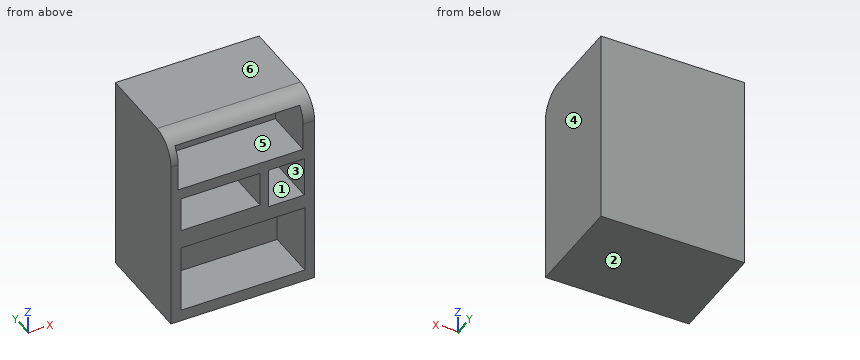
```python
from build123d import *

# Parameters (mm, degrees)
F0_W        = 71.2871104479
F0_H        = 49.0286853164
F0_W_2      = 58.531470614
F0_H_2      = 36.0211754636
F0_W_3      = 60.9135755652
F0_H_3      = 33.0608540971
F1_DEPTH    = 50.8
F2_W        = 39.112127386
F2_H        = 17.2953940928
F2_W_2      = 17.7711145952
F2_H_2      = 19.8306103703
F2_W_3      = 61.416560784
F2_H_3      = 33.9031042531
F2_W_4      = 61.9626361877
F2_H_4      = 21.9576358795
F3_DEPTH    = 25.4
F4_T1_DEPTH = 134.7871104479


# Not quite as in the source:
# - a fillet or chamfer that OpenCascade refuses, or shapes differently, is made with other operations: its cross-section is extruded or revolved along the edge and cut away or added


with BuildPart() as f1:
    # F0 (on Front) → F1 (new body)
    with BuildSketch(Plane.XZ):
        with Locations((0, 24.5143426582)):
            Rectangle(F0_W, F0_H)
        with Locations((-0.6145685997, 23.0905877318)):
            Rectangle(F0_W_2, F0_H_2, mode=Mode.SUBTRACT)
        with Locations((0, -24.5143426582)):
            Rectangle(F0_W, F0_H)
        with Locations((0.2925068763, -25.7660689676)):
            Rectangle(F0_W_3, F0_H_3, mode=Mode.SUBTRACT)
        with Locations((-0.6145685997, 23.0905877318)):
            Rectangle(F0_W_2, F0_H_2)
        with Locations((0.2925068763, -25.7660689676)):
            Rectangle(F0_W_3, F0_H_3)
    extrude(amount=F1_DEPTH)

    # F2 (on face) → F3 (cut)
    with BuildSketch(Plane.XZ.offset(50.8)):
        with Locations((-10.9740667976, 8.6476970464)):
            Rectangle(F2_W, F2_H)
        with Locations((21.669532638, 7.5109825702)):
            Rectangle(F2_W_2, F2_H_2)
        with Locations((0.1781499013, -26.3703963719)):
            Rectangle(F2_W_3, F2_H_3)
        with Locations((-1.0527623817, 33.6884222925)):
            Rectangle(F2_W_4, F2_H_4)
    extrude(amount=-F3_DEPTH, mode=Mode.SUBTRACT)

    # F4: fillet of radius 12.7 on 1 edges, made by hand

    # F4_s2 → F4_t1 (cut)
    with BuildSketch(Plane.YZ.offset(-67.3935552239)):
        with BuildLine():
            ThreePointArc((-50.8, 36.3286853164), (-47.0802561211, 45.3089414375), (-38.1, 49.0286853164))
            Line((-38.1, 49.0286853164), (-50.8, 49.0286853164))
            Line((-50.8, 49.0286853164), (-50.8, 36.3286853164))
        make_face()
    extrude(amount=F4_T1_DEPTH, mode=Mode.SUBTRACT)


solid = f1.part
```
Geometry: final body of the model. Coordinates: model frame, mm. Face numbers are marked on the shaded views. A direction names the side the tool comes from. Round coordinates to 2 decimals unless told otherwise and drop trailing zeros. Order: outer loops, then holes, each group sorted by start corner. A loop starts at its lowest first (then second) coordinate and runs counter-clockwise, first axis right, second up. Notation, with made-up numbers: (3, 3.25) -> (47, 3.25) arc R21 cw to (47, 22.25) -> close; hole circle Ø3 at (49.5, 83). An arc over 180 degrees is marked (long way). Use CSV: the item, a comma, the result in double quotes. Start each with the question number.
1) Section D-D (x = -1). Return the cut outline in (y, z), and give its area (3 significant figures).
2) First-contact query: pin 1 Ø4 at (x, z) = (5.5, 36) entering from -Y. Flat tip, straight axial feed; report the tip coordinate or a pass-through.
3) Section A-A (y = -33.5). Return the cut outline in (x, z), and give its area (3 significant figures).
4) Section B-B (x = 25). Return the cut outline in (y, z).
5) Set-up query: the marked faces 1 and 2. Return all of +Z, -Z, +X, -X, +Y, -Y with unobstructed straight access to the full face (end or side cutting, diameter ignored); none if empty.
6) Section C-C (z = -33.5). Return the cut outline in (x, y).
7) Material intervals for line 1 along Z through (x, y) = (-4, -33); line 2 along X through (y, z) = (-28, 16.5); line 3 along Z through (x, y) = (-32, -31), sorted ascending. Write a range as from..to.
8) Draft query along X for the marked faces 3, 4, 5 and 6. Return one class per face: +X half, -X half, draft (parallel to the pull), parting line (faces both ways), or undercut.
Returned:
1,outline,"(-50.8, -49.03) -> (0, -49.03) -> (0, 49.03) -> (-38.1, 49.03) arc R12.7 ccw to (-47.68, 44.67) -> (-25.4, 44.67) -> (-25.4, 22.71) -> (-50.8, 22.71) -> (-50.8, 17.3) -> (-25.4, 17.3) -> (-25.4, 0) -> (-50.8, 0) -> (-50.8, -9.42) -> (-25.4, -9.42) -> (-25.4, -43.32) -> (-50.8, -43.32) -> close"
1,area,"3,100 mm²"
2,pin 1,"stops at y = -25.4"
3,outline,"(-35.64, -49.03) -> (35.64, -49.03) -> (35.64, 49.03) -> (-35.64, 49.03) -> close; hole (-32.03, 22.71) -> (29.93, 22.71) -> (29.93, 44.67) -> (-32.03, 44.67) -> close; hole (-30.53, -43.32) -> (30.89, -43.32) -> (30.89, -9.42) -> (-30.53, -9.42) -> close; hole (-30.53, 0) -> (8.58, 0) -> (8.58, 17.3) -> (-30.53, 17.3) -> close; hole (12.78, -2.4) -> (30.56, -2.4) -> (30.56, 17.43) -> (12.78, 17.43) -> close"
3,area,"2,520 mm²"
4,outline,"(-50.8, -49.03) -> (0, -49.03) -> (0, 49.03) -> (-38.1, 49.03) arc R12.7 ccw to (-47.68, 44.67) -> (-25.4, 44.67) -> (-25.4, 22.71) -> (-50.8, 22.71) -> (-50.8, 17.43) -> (-25.4, 17.43) -> (-25.4, -2.4) -> (-50.8, -2.4) -> (-50.8, -9.42) -> (-25.4, -9.42) -> (-25.4, -43.32) -> (-50.8, -43.32) -> close"
5,face 1,"-Y"
5,face 2,"-Z, +X, -X, +Y, -Y"
6,outline,"(-35.64, -50.8) -> (-30.53, -50.8) -> (-30.53, -25.4) -> (30.89, -25.4) -> (30.89, -50.8) -> (35.64, -50.8) -> (35.64, 0) -> (-35.64, 0) -> close"
7,line 1,"z = -49.03..-43.32, -9.42..0, 17.3..22.71, 44.67..49.03"
7,line 2,"x = -35.64..-30.53, 8.58..12.78, 30.56..35.64"
7,line 3,"z = -49.03..22.71, 44.67..49.03"
8,face 3,"undercut"
8,face 4,"+X half"
8,face 5,"undercut"
8,face 6,"draft"
